Geometry check sheet. Reference: the model listing, model coordinates, mm. A direction names the side the tool comes from. Round coordinates to 2 decimals unless told otherwise and drop trailing zeros. Write each loop counter-clockwise with the first axis right and the second up, starting at its lowest first coordinate (ties: lowest second). Pieces come first, ordered by that corner, then holes. Notation, with made-up numbers: (12.5, 36) - (46.5, 36) arc R18 cw to (46.5, 69) - close; hole circle Ø4 at (-4.75, 58). An arc over 180 degrees is marked (long way). Return JSON: item names as keys, results as strings. Group by question number.
Autodesk Inventor part; units mm, degrees
ref_plane "YZ Plane" through (0, 0, 0) normal (1, 0, 0) x (0, 1, 0)
ref_plane "XZ Plane" through (0, 0, 0) normal (0, 1, 0) x (-1, 0, 0)
ref_plane "XY Plane" through (0, 0, 0) normal (0, 0, 1) x (1, 0, 0)
sketch "Skizze1" plane through (0, 0, 0) normal (0, 1, 0) x (-1, 0, 0)
  line L0 (0, 82.3152) -> (0, -45.1122)
  line L1 (250, 500) -> (250, 0)
  line L2 (250, 0) -> (250, 0)
  line L3 (250, 0) -> (100, -116.2752)
  line L4 (100, -116.2752) -> (100, -122.6015)
  line L5 (100, -122.6015) -> (251.711, -5)
  line L6 (251.711, -5) -> (255, -5)
  line L7 (255, -5) -> (255, 500)
  line L8 (255, 500) -> (250, 500)
  line L9 (306, 0) -> (-51, 0)
  point P0 (0, 0)
  dimension "d0" = 5
  dimension "d1" = 5
  dimension "d2" = 5
  dimension "d3" = 500
  dimension "d4" = 500
  dimension "d5" = 500
  dimension "d6" = 200
revolve "Umdrehung1" add sketch "Skizze1" angle 360 about axis through (0, 0, 82.3152) along (0, 0, -1)
sketch "Skizze3" plane through (0, 0, 0) normal (0, 1, 0) x (-1, 0, 0)
  line L0 (-251.711, -5) -> (-100, -122.6015)
  line L1 (-397.6603, 108.1352) -> (-63.9838, -150.52)
  point P0 (0, 0)
ref_plane "Arbeitsebene1" through (397.6603, 0, 108.1352) normal (-0.6127, 0, 0.7904) x (0, -1, 0)
sketch "Skizze4" plane through (397.6603, 0, 108.1352) normal (-0.6127, 0, 0.7904) x (0, -1, 0)
  circle A0 centre (0, -278.6039) radius 90
  ellipse E0 centre (0, -383.6039) end of major axis (251.711, -383.6039) minor radius 198.94
  point P0 (0, -380.5407)
  dimension "d12" = 180
  dimension "d13" = 105
extrude "Extrusion2" add sketch "Skizze4" along normal up to surface contours A0
sketch "Skizze5" plane through (397.6603, 0, 108.1352) normal (0.6127, 0, -0.7904) x (-0.7904, 0, -0.6127)
  circle A0 centre (278.6039, 0) radius 85
  arc A1 (368.6039, 0) -> (188.6039, 0) centre (278.6039, 0) ccw
  point P0 (380.5407, 0)
  dimension "d16" = 170
extrude "Extrusion3" cut sketch "Skizze5" against normal up to surface
equation "\"d1\" = d0"
equation "\"d2\" = d0"
properties part number "Tank_1"
1. Section check C-C (z = 292). Enter the section's corners in (x, y).
2. Material ranges on line 1 along Y through (x, z) = (0, 120); line 2 along X through (y, z) = (-9, 52.5); line 3 along X through (y, z) = (2, 459.5), recorded low to high.
3. Section check A-A (x = 0). Enter the section's corners in (y, z).
4. Tool access check on faces 1 (the face through (-188, -169, -5)), 2 (the face through (-104.33, -32.86, -109)). Record the directions out of +Z, -Z, +X, -X, +Y, -Y that give a thin tool (end or side, any length) a straight path to the whole face; none if there is none.
5. Mould release check, pull along X, two halves, no side actions. Record for faces 3 (the face through (249.76, 10.99, 246.5)), 4 (the face through (114.136, -48.383, -104.723)), 5 (the face through (-188, -169, 500)), 6 (the face through (55, 249, 251)): pulls with the +X half, pulls with the -X half, needs draft (parallel to the pull), parting line crosses it, or undercut.
6. Depth check by flat-ended pin: pin 1 Ø6 at (x, z) = (111, 287.5) entering from +Y; pin 2 Ø5 at (x, y) = (4, -133.5) entering from +Z; pin 3 Ø5 at (x, z) = (138.5, -21.5) entering from -Y. Enter the tip coordinate at first touch or a pass-through.
7. Section check B-B (y = 0). State how many separate pieces and enclosed holes the cut face has, and give its area (3 significant figures).
Result sheet:
{
 "1": {"outline": "circle Ø510 at (0, 0); hole circle Ø500 at (0, 0)"},
 "2": {"line 1": "y = -255 to -250, 250 to 255", "line 2": "x = -254.84 to -249.84, 249.84 to 254.84", "line 3": "x = -254.99 to -249.99, 249.99 to 254.99"},
 "3": {"outline": "(-255, -5) - (-251.71, -5) - (-100, -122.6) - (-100, -116.28) - (-250, 0) - (-250, 500) - (-255, 500) - close; (100, -122.6) - (251.71, -5) - (255, -5) - (255, 500) - (250, 500) - (250, 0) - (100, -116.28) - close"},
 "4": {"face 1": "-Z", "face 2": "+Z"},
 "5": {"face 3": "undercut", "face 4": "undercut", "face 5": "needs draft", "face 6": "parting line crosses it"},
 "6": {"pin 1": "stops at y = 231", "pin 2": "stops at z = -88.32", "pin 3": "stops at y = -188.58"},
 "7": {"separate pieces": "3", "enclosed holes": "0", "area": "6,100 mm²"}
}
